CAD build for the part. Positions are in the model's coordinates, mm. Face numbers are marked on the shaded views. Give positions to 0.01 mm unless a question says otherwise; leave off trailing zeros. One line per question, with ' | ' between items.
```python
from build123d import *

# Parameters (mm, degrees)
ESQUISSE3_R             = 1.75
ENL_V_MAT_EXTRU_1_DEPTH = 0.5
ENL_V_MAT_EXTRU_1_DRAFT = -16
CONG_1_R                = 0.25


with BuildPart() as part:
    # Esquisse1 → Base-Révolution (revolve)
    with BuildSketch(Plane.XY):
        Polygon((-3.671011888, 20.208682969), (-13.724147668, 17.415887566), (-13.132038717, 14.901290759), (-2.868011513, 17.318148347), align=None)
    revolve(axis=Axis((5.13679497, 22.65552175, 0), (-0.9635115404771745, -0.2676667916782024, 0)))


with BuildPart() as enl_v_mat_extru_1_tool:
    # Esquisse3 → Enlèv. mat.-Extru.1 (with draft: the straight prism first)
    with BuildSketch(Plane(origin=(1.80645753, 0.491612486, 0), x_dir=(0, 0, -1), z_dir=(0.9635115404771745, 0.2676667916782024, 0))):
        with Locations((0, 20.463761621)):
            Circle(ESQUISSE3_R)
    extrude(amount=-ENL_V_MAT_EXTRU_1_DEPTH)
    # Enlèv. mat.-Extru.1: the draft: its side faces are tilted about the plane it starts from
    enl_v_mat_extru_1_sides = [enl_v_mat_extru_1_tool.faces().sort_by_distance(p)[0] for p in [
        (-3.911889774, 20.141766271, 1.75),
    ]]
    draft(enl_v_mat_extru_1_sides, Plane(origin=(1.80645753, 0.491612486, 0), x_dir=(0, 0, -1), z_dir=(0.9635115404771745, 0.2676667916782024, 0)), ENL_V_MAT_EXTRU_1_DRAFT)


with BuildPart() as part_1:
    add(part.part)

    # Enlèv. mat.-Extru.1: cut by enl_v_mat_extru_1_tool
    add(enl_v_mat_extru_1_tool.part, mode=Mode.SUBTRACT)

    # Congé1
    cong_1_edges = [part_1.edges().sort_by_distance(p)[0] for p in [
        (-14.513911863, 19.875575073, 0),
        (-4.474012264, 23.09921759, 0),
    ]]
    fillet(cong_1_edges, radius=CONG_1_R)


solid = part_1.part
```
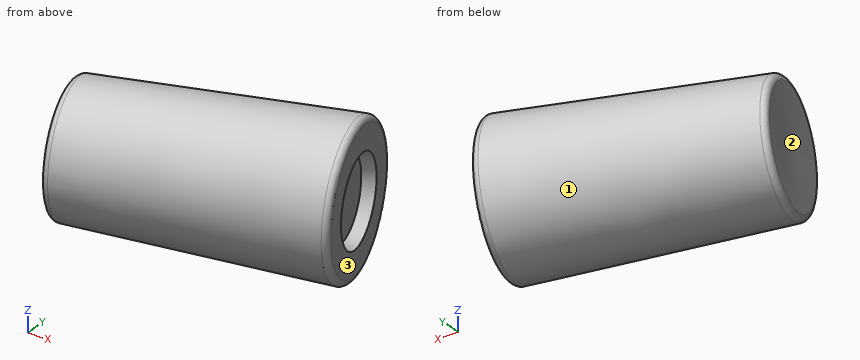
Item 1: Drill centre lines: line 1 along Y through (x, z) = (-12.75, -2.25); line 2 along Y through (x, z) = (-8.75, 1.25); line 3 along X through (y, z) = (18.5, -1.9). Where is each one in solid material? Low to high. Write a range as [from, to].
Conclusion:
line 1: [16.31, 19.12] | line 2: [16.24, 21.42] | line 3: [-14.12, -3.2]
Item 2: Drop flat-ended pins along their axis: P1, Ø1.5, axis at x = -12.5, y = 20.5, coming from the +Z side; P2, Ø1.5, axis at x = -10.5, y = 20, coming from the +Z side; P3, Ø2, axis at x = -4, z = -0.5, coming from the -Y side. Give the stop position or say it passes through.
Conclusion:
P1: z = 1.88 | P2: z = 2.59 | P3: y = 16.83
Item 3: Mould opens along Z. For the marked faces 1, 2 and 3 say: pulls with the +Z half, pulls with the -Z half, needs draft (parallel to the pull), parting line crosses it, or undercut.
Conclusion:
face 1: parting line crosses it | face 2: undercut | face 3: needs draft
